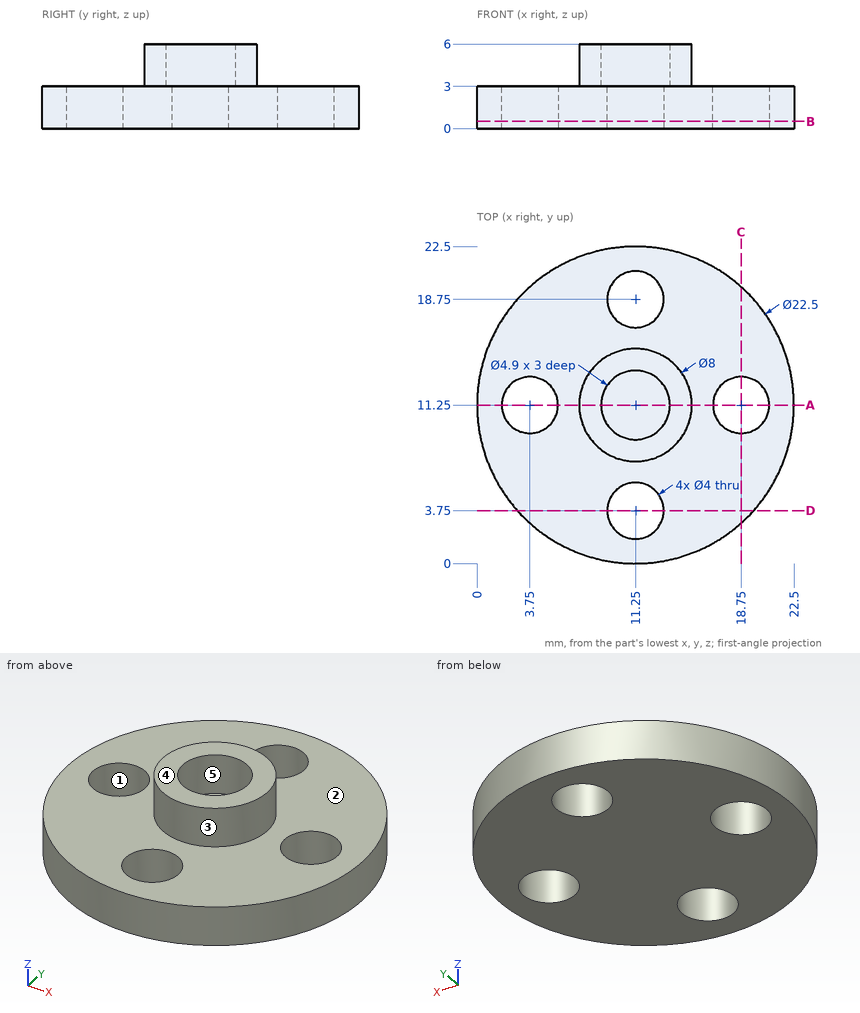
Drawing for the job (mm, zero at the part's lowest x, y, z). A direction names the side the tool comes from. Round coordinates to 2 decimals unless told otherwise and drop trailing zeros. Order: outer loops, then holes, each group sorted by start corner. A loop starts at its lowest first (then second) coordinate and runs counter-clockwise, first axis right, second up.
Item 1: Pin check, flat tips, straight feed: pin 1 (3 mm diameter, centred on x = 11.25, y = 18.75, fed in from +Z); pin 2 (5.5 mm diameter, centred on x = 12, y = 11.5, fed in from +Z); pin 3 (3 mm diameter, centred on x = 11.25, y = 11.25, fed in from +Z); pin 4 (1 mm diameter, centred on x = 13.5, z = 2, fed in from -Y). Stop position of each tip, or through.
Item 2: Saw through at C-C on x = 18.75. Write the cut outline in (y, z), then the cut area to 3 significant figures.
Item 3: Mould opens along Y. For the marked faces 1, 2 and 3 say: pulls with the +Y half, pulls with the -Y half, needs draft (parallel to the pull), parting line crosses it, or undercut.
Item 4: Saw through at A-A on y = 11.25. Write the cut outline in (x, z).
Item 5: Tool access for the marked faces 4 and 5: list every direction of +Z, -Z, +X, -X, +Y, -Y with a clear straight run to the whole face (end or side of a thin tool).
Item 6: Saw through at B-B on z = 0.5. Write the cut outline in (x, y).
Item 7: Probe line 1 along Y through (x, z) = (11.25, 2.3); line 2 along Z through (x, y) = (9, 6.5); line 3 along Y through (x, z) = (18.75, 1.9). List the from-to ranges inside material, lowest first.
Reported:
1. pin 1: passes through
1. pin 2: stops at z = 6
1. pin 3: stops at z = 3
1. pin 4: stops at y = 0.14
2. outline: (2.86, 0) - (9.25, 0) - (9.25, 3) - (2.86, 3) - close; (13.25, 0) - (19.64, 0) - (19.64, 3) - (13.25, 3) - close
2. area: 38.3 mm2
3. face 1: undercut
3. face 2: needs draft
3. face 3: parting line crosses it
4. outline: (0, 0) - (1.75, 0) - (1.75, 3) - (0, 3) - close; (5.75, 0) - (16.75, 0) - (16.75, 3) - (15.25, 3) - (15.25, 6) - (13.7, 6) - (13.7, 3) - (8.8, 3) - (8.8, 6) - (7.25, 6) - (7.25, 3) - (5.75, 3) - close; (20.75, 0) - (22.5, 0) - (22.5, 3) - (20.75, 3) - close
5. face 4: +Z, +X, -X, +Y, -Y
5. face 5: +Z
6. outline: circle Ø22.5 at (11.25, 11.25); hole circle Ø4 at (3.75, 11.25); hole circle Ø4 at (11.25, 3.75); hole circle Ø4 at (11.25, 18.75); hole circle Ø4 at (18.75, 11.25)
7. line 1: y = 0 to 1.75, 5.75 to 16.75, 20.75 to 22.5
7. line 2: z = 0 to 3
7. line 3: y = 2.86 to 9.25, 13.25 to 19.64
